```python
from build123d import *

# Parameters (mm, degrees)
F1_W     = 131.9631
F1_H     = 51.463606
F2_DEPTH = 20.32
F3_DEPTH = 20.32
F4_DEPTH = 57.15


with BuildPart() as f2:
    # F1 (on Top) → F2 (new body)
    with BuildSketch(Plane.XY):
        with Locations((-32.353217, -2.002475)):
            Rectangle(F1_W, F1_H)
    extrude(amount=F2_DEPTH)

    # F0 (on Top) → F3 (join)
    with BuildSketch(Plane.XY):
        with BuildLine():
            ThreePointArc((-69.85, 0), (-91.530256, 8.980256), (-82.55, -12.7))
            ThreePointArc((-82.55, -12.7), (-73.569744, -8.980256), (-69.85, 0))
        make_face()
        Polygon((-41.275, -9.525), (-31.75, -9.525), (-22.225, -9.525), (-22.225, 9.525), (-41.275, 9.525), align=None)
    extrude(amount=-F3_DEPTH)

    # F0 (on Top) → F4 (cut)
    with BuildSketch(Plane.XY):
        Polygon((19.05, -21.997045), (6.35, 0), (-6.35, -21.997045), align=None)
    extrude(amount=F4_DEPTH, mode=Mode.SUBTRACT)


solid = f2.part
```
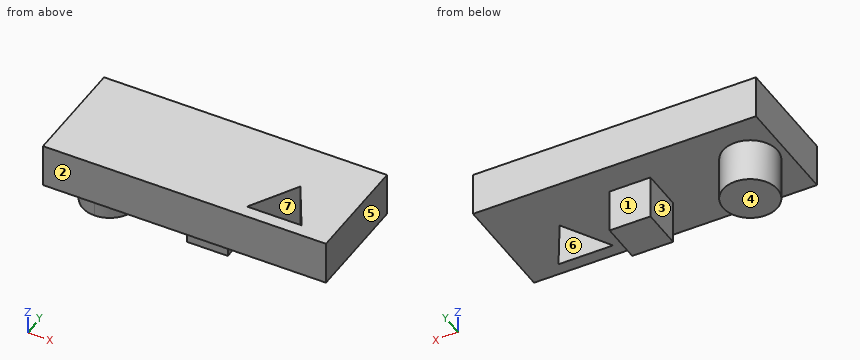
Can you work these out from the model? Positions are in its coordinate system, mm. Face numbers are marked on the shaded views. A direction names the side the tool comes from. Round coordinates to 2 decimals unless told otherwise and drop trailing zeros. Loops run counter-clockwise (first coordinate to the right, second up) from the corner with the lowest first, then second, coordinate; pieces in that order, holes last.
Item 1: Will these pins go through, and if not, where does the flat tip stop? pin 1 Ø9.5 at (y, z) = (1.5, -13.5) entering from -X; pin 2 Ø9.5 at (x, z) = (-29, -7) entering from +Y (3 decimals); pin 3 Ø1 at (x, y) = (-73, -14) entering from -Z.
Item 2: Suppose I cut it at D-D, the plane y = -17.5. Write out the boundary of the cut face in (x, z).
Item 3: Suppose I cut it at A-A, the plane z = 6. Write out the boundary of the cut face in (x, y).
Item 4: Please list where these lines run through material, in increasing order: L1, parallel to Z at x = 1.5, y = 8.5; L2, parallel to Y at x = 4.5, z = 2; L3, parallel to X at y = -18, z = 13.5.
Item 5: Which directions (+Z, -Z, +X, -X, +Y, -Y) give clear straight access to the entire face, cutting with the end or side of a thin tool? Please do the marked faces 1, 2 and 3.
Item 6: Suppose I cut it at C-C, the plane x = -27.5. Write out the boundary of the cut face in (y, z) (3 decimals), then the cut area to 3 significant figures.
Item 7: Suppose I cut it at B-B, the plane z = -12. Write out the boundary of the cut face in (x, y) (3 decimals).
Item 8: If we mould it in two halves opening along X, with no side actions, what happens to the marked faces 4, 5, 6 and 7? For each: +X half, -X half, draft (parallel to the pull), parting line (faces both ways), or undercut.
Reported:
1. pin 1: stops at x = -95.25
1. pin 2: stops at y = 9.525
1. pin 3: stops at z = 0
2. outline: (-98.33, 0) - (-3.75, 0) - (-3.75, 20.32) - (-98.33, 20.32) - close; (16.45, 0) - (33.63, 0) - (33.63, 20.32) - (16.45, 20.32) - close
3. outline: (-98.33, -27.73) - (33.63, -27.73) - (33.63, 23.73) - (-98.33, 23.73) - close; hole (-6.35, -22) - (19.05, -22) - (6.35, 0) - close
4. L1: z = 0 to 20.32
4. L2: y = -27.73 to -22, -3.2 to 23.73
4. L3: x = -98.33 to -4.04, 16.74 to 33.63
5. face 1: -Z, +X, +Y
5. face 2: +Z, -Z, +X, -X, -Y
5. face 3: -Z, +Y, -Y
6. outline: (-27.734, 0) - (-9.525, 0) - (-9.525, -20.32) - (9.525, -20.32) - (9.525, 0) - (23.729, 0) - (23.729, 20.32) - (-27.734, 20.32) - close
6. area: 1,430 mm2
7. outline: circle Ø25.4 at (-82.55, 0); (-41.275, -9.525) - (-22.225, -9.525) - (-22.225, 9.525) - (-41.275, 9.525) - close
8. face 4: draft
8. face 5: +X half
8. face 6: undercut
8. face 7: undercut
